from build123d import *

# Parameters (mm, degrees)
BOSS_EXTRUDE1_DEPTH = 18.4
SKETCH2_R           = 5
BOSS_EXTRUDE2_DEPTH = 20
DOME1_FACE_RADIUS   = 5
DOME1_HEIGHT        = 1
SKETCH3_R           = 1
BOSS_EXTRUDE3_DEPTH = 40
BOSS_EXTRUDE4_START = -15
SKETCH4_R           = 2.5
BOSS_EXTRUDE4_DEPTH = 18
FILLET1_R           = 5


with BuildPart() as part:
    # Sketch1 → Boss-Extrude1 (new body)
    with BuildSketch(Plane.XY):
        with BuildLine():
            Line((-17.563883718, 9.91167305), (-1.563883718, 9.91167305))
            add(Edge.make_bspline(
                [(-1.563883718, 9.91167305), (4.3404042, 0.119497618), (-1.563883718, -11.08832695)],
                knots=[0, 0, 0, 1, 1, 1], degree=2))
            Line((-1.563883718, -11.08832695), (-17.563883718, -11.08832695))
            Line((-17.563883718, -11.08832695), (-17.563883718, 9.91167305))
        make_face()
    extrude(amount=BOSS_EXTRUDE1_DEPTH)

    # Sketch2 → Boss-Extrude2 (add)
    with BuildSketch(Plane.ZY.offset(17.563883718)):
        with Locations((9.2, -0.58832695)):
            Circle(SKETCH2_R)
    extrude(amount=-BOSS_EXTRUDE2_DEPTH)

    # Dome1: a dome of height H over a round flat face of radius A is a cap of a sphere of radius (A * A + H * H) / (2 * H)
    dome1_r = (DOME1_FACE_RADIUS * DOME1_FACE_RADIUS + DOME1_HEIGHT * DOME1_HEIGHT) / (2 * DOME1_HEIGHT)
    dome1_base = Plane((2.436116282, -0.58832695, 9.2), z_dir=(1, 0, 0))
    with Locations(dome1_base.offset(DOME1_HEIGHT - dome1_r)):
        dome1_ball = Sphere(dome1_r, mode=Mode.PRIVATE)
    add(split(dome1_ball, bisect_by=dome1_base, keep=Keep.TOP, mode=Mode.PRIVATE))

    # Sketch3 → Boss-Extrude3 (add)
    with BuildSketch(Plane(origin=(0, 9.91167305, 0), x_dir=(1, 0, 0), z_dir=(0, 1, 0))):
        with Locations(Location((-16.067507499, -9.2, 0), (0, 0, 90))):
            Circle(SKETCH3_R)
    extrude(amount=BOSS_EXTRUDE3_DEPTH)

    # Sketch4 → Boss-Extrude4 (add)
    with BuildSketch(Plane(origin=(0, 49.91167305, 0), x_dir=(1, 0, 0), z_dir=(0, 1, 0)).offset(BOSS_EXTRUDE4_START)):
        with Locations(Location((-16.067507499, -9.2, 0), (0, 0, 270))):
            Circle(SKETCH4_R)
    extrude(amount=-BOSS_EXTRUDE4_DEPTH)

    # Fillet1
    # the kernel refuses this fillet: 5 mm, written as the material it adds along each edge
    with BuildSketch(Plane(origin=(-16.067507499, 34.91167305, 9.2), x_dir=(0, 0, -1), z_dir=(-1, 0, 0))) as fillet1_piece_1:
        with BuildLine():
            CenterArc((6, -3.570714214), FILLET1_R, 134.427004001, 45.572995999)
            Line((1, -3.570714214), (0.9, -3.570714214))
            Line((0.9, -3.570714214), (0.9, 0))
            Line((0.9, 0), (1, 0.1))
            ThreePointArc((1, 0.1), (1.75, 0.1), (2.43, 0.071414284))
            Line((2.43, 0.071414284), (2.5, 0))
        make_face()
    revolve(axis=Axis((-16.067507499, 34.91167305, 9.2), (0, -1, 0)))


solid = part.part
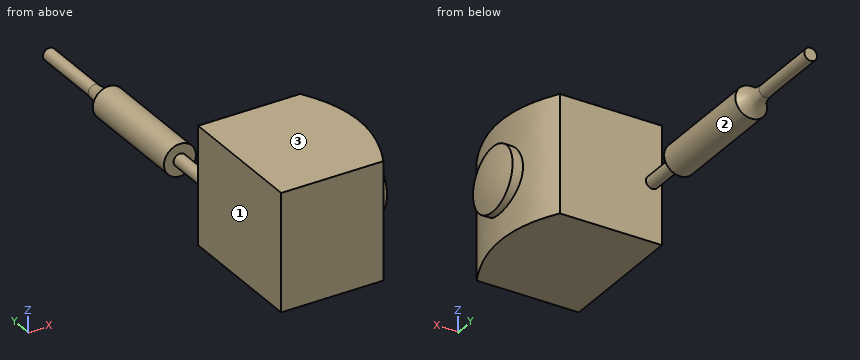
Check sheet for the modelled part. Datum: model origin and axes. Units: mm. Face numbers are marked on the shaded views. A direction names the side the tool comes from. Give positions to 0.01 mm unless a question says otherwise; leave off trailing zeros. Write each loop counter-clockwise with the first axis right and the second up, starting at its lowest first coordinate (ties: lowest second). Pieces come first, ordered by that corner, then holes. Notation, with made-up numbers: (14, 64.25) -> (51, 64.25) arc R22 ccw to (51, 72.25) -> close; hole circle Ø4 at (56.25, -37). An arc over 180 degrees is marked (long way). One line per item, written item: value. Start each with the question number.
Item 1: Material ranges on probe 1 along Y at (x, z) = (-15.5, 17.25); probe 2 along X at (y, z) = (33, 8.5); probe 3 along Y at (x, z) = (2.25, 8.5), recorded low to high. Write a range as from..to.
Item 2: Tool access check on the marked faces 1, 2 and 3. Record the directions out of +Z, -Z, +X, -X, +Y, -Y that give a thin tool (end or side, any length) a straight path to the whole face; none if there is none.
Item 3: Section check A-A on x = -6. Record the cut outline in (y, z), then the cut area to 3 significant figures.
Item 4: Gauge pin test, flat ends, axial feed: pin 1 (5 mm diameter, centred on x = -7.5, z = 6.5, fed in from +Y); pin 2 (4 mm diameter, centred on y = 33.5, z = 9.5, fed in from +X); pin 3 (10 mm diameter, centred on x = -12, y = 37, fed in from +Z). Record the tip position at first contact, or that the pin passes through.
Results list:
1. probe 1: -11.09..9.91
1. probe 2: -18.47..-13.67
1. probe 3: -5.54..4.36
2. face 1: +Z, -Z, -X, -Y
2. face 2: +Y
2. face 3: +Z, +X, -X, +Y, -Y
3. outline: (-11.09, 0) -> (9.91, 0) -> (9.91, 18.4) -> (-11.09, 18.4) -> close
3. area: 386 mm²
4. pin 1: y = 9.91
4. pin 2: x = -13.57
4. pin 3: z = 11.7
